The listing builds one solid part. Answer for the finished solid, in the listing's coordinates (mm). Face numbers are marked on the shaded views. A direction names the side the tool comes from. Give positions to 0.01 mm unless a question says otherwise; leave off trailing zeros. Loops run counter-clockwise (first coordinate to the right, second up) from the corner with the lowest first, then second, coordinate; pieces in that order, holes last. Notation, with made-up numbers: M 81,37.5 L 132,37.5 A27 cw 132,56.5 Z; hole C 12.25,-37 d11. An arc over 180 degrees is marked long. One line per item, written item: value. Start each with the question number.
Q1. Consider L1, parallel to Z at x = 50, y = 8.7 (3 decimals); L2, parallel to Z at x = 8.95, y = 1.5; L3, parallel to Z at x = 71.05, y = 10. Determine where each line is inside the solid, lowest interval first.
Q2. A cutting plane is placed at D-D, the plane y = -11. Determine the outline of the cut face in (x, z) (3 decimals), and give its area (3 significant figures).
Q3. A cutting plane is placed at A-A, the plane x = 28.95. Determine the outline of the cut face in (y, z).
Q4. Flat-ended cylindrical pins translate along their axes: pin 1 (8 mm diameter, centred on y = 12, z = -65.5, fed in from +X); pin 2 (3 mm diameter, centred on x = 37.5, z = -115, fed in from -Y); pin 3 (9.5 mm diameter, centred on y = 3, z = -75, fed in from -X); pin 4 (5 mm diameter, centred on x = 83, z = -26.5, fed in from -Y). Find the tip coordinate at first contact, or state that the pin passes through.
Q5. A cutting plane is placed at B-B, the plane z = -56.47. Determine the outline of the cut face in (x, y).
Q6. A cutting plane is placed at C-C, the plane z = -92. Determine the outline of the cut face in (x, y), and give its area (3 significant figures).
Q7. For the marked faces 1, 2 and 3, determine the directions among +Z, -Z, +X, -X, +Y, -Y from which every point of the face is accessible in a straight line to the end or side of a thin tool.
from build123d import *

# Parameters (mm, degrees)
SKETCH1_W                      = 100
SKETCH1_H                      = 37
BOSS_EXTRUDE1_DEPTH            = 6
M3_CLEARANCE_HOLE1_D           = 3.4
SKETCH31_W                     = 20
SKETCH31_H                     = 29.63
BOSS_EXTRUDE9_DEPTH            = 16
BOSS_EXTRUDE9_DEPTH_BACK       = 9
SKETCH32_W                     = 100
SKETCH32_H                     = 5
BOSS_EXTRUDE10_DEPTH           = 16
SKETCH33_R                     = 3
BOSS_EXTRUDE11_DEPTH           = 3
SKETCH34_W                     = 3
SKETCH34_H                     = 19.5
CUT_EXTRUDE1_DEPTH             = 101
CUT_EXTRUDE2_START             = -2.5
SKETCH35_W                     = 20
SKETCH35_H                     = 20.32
CUT_EXTRUDE2_DEPTH             = 19.5
SKETCH36_R                     = 2.5
CUT_EXTRUDE3_DEPTH             = 26
FILLET1_R                      = 5
SKETCH37_R                     = 3
SKETCH37_R_2                   = 2.5
BOSS_EXTRUDE12_DEPTH           = 6.5
BOSS_EXTRUDE12_DEPTH_BACK      = 2.5
CBORE_FOR_M5_SHCS1_D           = 5.5
CBORE_FOR_M5_SHCS1_CBORE_D     = 10
CBORE_FOR_M5_SHCS1_CBORE_DEPTH = 26
M5_CLEARANCE_HOLE1_D           = 5.5
FILLET3_R                      = 5
SKETCH48_W                     = 11.20158878
SKETCH48_H                     = 10
BOSS_EXTRUDE15_DEPTH           = 14


with BuildPart() as part:
    # Sketch1 → Boss-Extrude1 (new body)
    with BuildSketch(Plane(origin=(0, 0, 0), x_dir=(1, 0, 0), z_dir=(0, 1, 0))):
        with Locations((50, 18.5)):
            Rectangle(SKETCH1_W, SKETCH1_H)
    extrude(amount=BOSS_EXTRUDE1_DEPTH)

    # M3 Clearance Hole1 (through all)
    with Locations(Plane(origin=(0, 0, 0), x_dir=(-1, 0, 0), z_dir=(0, -1, 0))):
        with Locations((-8.95, 3.5), (-8.95, 28.5), (-28.95, 28.5), (-28.95, 3.5), (-71.05, 3.5), (-71.05, 28.5), (-91.05, 28.5), (-91.05, 3.5)):
            Hole(M3_CLEARANCE_HOLE1_D / 2)

    # Sketch31 → Boss-Extrude9 (add, two sides)
    with BuildSketch(Plane.XZ) as boss_extrude9_sk:
        with Locations((50, -51.815)):
            Rectangle(SKETCH31_W, SKETCH31_H)
    extrude(amount=BOSS_EXTRUDE9_DEPTH)
    extrude(boss_extrude9_sk.sketch, amount=-BOSS_EXTRUDE9_DEPTH_BACK)

    # Sketch32 → Boss-Extrude10 (add)
    with BuildSketch(Plane.XZ):
        with Locations((50, -34.5)):
            Rectangle(SKETCH32_W, SKETCH32_H)
    extrude(amount=BOSS_EXTRUDE10_DEPTH)

    # Sketch33 → Boss-Extrude11 (add)
    with BuildSketch(Plane(origin=(0, 6, 0), x_dir=(1, 0, 0), z_dir=(0, 1, 0))):
        Polygon((0, 37), (0, 0), (100, 0), (100, 37), (60, 37), (40, 37), align=None)
        with Locations((71.05, 3.5)):
            Circle(SKETCH33_R, mode=Mode.SUBTRACT)
        with Locations((71.05, 28.5)):
            Circle(SKETCH33_R, mode=Mode.SUBTRACT)
        with Locations((28.95, 3.5)):
            Circle(SKETCH33_R, mode=Mode.SUBTRACT)
        with Locations((28.95, 28.5)):
            Circle(SKETCH33_R, mode=Mode.SUBTRACT)
        with Locations((8.95, 28.5)):
            Circle(SKETCH33_R, mode=Mode.SUBTRACT)
        with Locations((8.95, 3.5)):
            Circle(SKETCH33_R, mode=Mode.SUBTRACT)
        with Locations((91.05, 3.5)):
            Circle(SKETCH33_R, mode=Mode.SUBTRACT)
        with Locations((91.05, 28.5)):
            Circle(SKETCH33_R, mode=Mode.SUBTRACT)
    extrude(amount=BOSS_EXTRUDE11_DEPTH)

    # Sketch34 → Cut-Extrude1 (cut, through all)
    with BuildSketch(Plane(origin=(100, 0, 0), x_dir=(0, 0, -1), z_dir=(1, 0, 0))):
        with Locations((37.5, -3.25)):
            Rectangle(SKETCH34_W, SKETCH34_H)
    extrude(amount=-CUT_EXTRUDE1_DEPTH, mode=Mode.SUBTRACT)

    # Sketch35 → Cut-Extrude2 (cut)
    with BuildSketch(Plane(origin=(0, 9, 0), x_dir=(1, 0, 0), z_dir=(0, 1, 0)).offset(CUT_EXTRUDE2_START)):
        with Locations((50, 56.47)):
            Rectangle(SKETCH35_W, SKETCH35_H)
    extrude(amount=-CUT_EXTRUDE2_DEPTH, mode=Mode.SUBTRACT)

    # Sketch36 → Cut-Extrude3 (cut, through all)
    with BuildSketch(Plane(origin=(0, 9, 0), x_dir=(1, 0, 0), z_dir=(0, 1, 0))):
        with Locations((50, 56.47)):
            Circle(SKETCH36_R)
    extrude(amount=-CUT_EXTRUDE3_DEPTH, mode=Mode.SUBTRACT)

    # Fillet1
    fillet1_edges = [part.edges().sort_by_distance(p)[0] for p in [
        (60, 7.75, -66.63),
        (40, 7.75, -66.63),
        (40, -14.5, -66.63),
        (60, -14.5, -66.63),
    ]]
    fillet(fillet1_edges, radius=FILLET1_R)

    # Sketch37 → Boss-Extrude12 (add, two sides)
    with BuildSketch(Plane(origin=(0, 9, 0), x_dir=(1, 0, 0), z_dir=(0, 1, 0))) as boss_extrude12_sk:
        Polygon((40, 37), (0, 37), (0, 0), (100, 0), (100, 37), (60, 37), (60, 137), (40, 137), align=None)
        with Locations((28.95, 3.5)):
            Circle(SKETCH37_R, mode=Mode.SUBTRACT)
        with Locations((8.95, 3.5)):
            Circle(SKETCH37_R, mode=Mode.SUBTRACT)
        with Locations((8.95, 28.5)):
            Circle(SKETCH37_R, mode=Mode.SUBTRACT)
        with Locations((28.95, 28.5)):
            Circle(SKETCH37_R, mode=Mode.SUBTRACT)
        with Locations((71.05, 28.5)):
            Circle(SKETCH37_R, mode=Mode.SUBTRACT)
        with Locations((91.05, 28.5)):
            Circle(SKETCH37_R, mode=Mode.SUBTRACT)
        with Locations((91.05, 3.5)):
            Circle(SKETCH37_R, mode=Mode.SUBTRACT)
        with Locations((71.05, 3.5)):
            Circle(SKETCH37_R, mode=Mode.SUBTRACT)
        with Locations((50, 56.47)):
            Circle(SKETCH37_R_2, mode=Mode.SUBTRACT)
    extrude(amount=BOSS_EXTRUDE12_DEPTH)
    extrude(boss_extrude12_sk.sketch, amount=-BOSS_EXTRUDE12_DEPTH_BACK)

    # CBORE for M5 SHCS1 (through all)
    with Locations(Plane(origin=(0, -16, 0), x_dir=(-1, 0, 0), z_dir=(0, -1, 0))):
        with Locations((-50, 127), (-50, 92)):
            CounterBoreHole(CBORE_FOR_M5_SHCS1_D / 2, CBORE_FOR_M5_SHCS1_CBORE_D / 2, CBORE_FOR_M5_SHCS1_CBORE_DEPTH)

    # M5 Clearance Hole1 (through all)
    with Locations(Plane(origin=(0, -16, 0), x_dir=(-1, 0, 0), z_dir=(0, -1, 0))):
        with Locations((-50, 42.655)):
            Hole(M5_CLEARANCE_HOLE1_D / 2)

    # Fillet3
    fillet3_edges = [part.edges().sort_by_distance(p)[0] for p in [
        (60, 11, -137),
        (40, 11, -137),
    ]]
    fillet(fillet3_edges, radius=FILLET3_R)

    # Sketch48 → Boss-Extrude15 (add)
    with BuildSketch(Plane.XZ):
        with Locations((50, -31)):
            Rectangle(SKETCH48_W, SKETCH48_H)
    extrude(amount=BOSS_EXTRUDE15_DEPTH)


solid = part.part
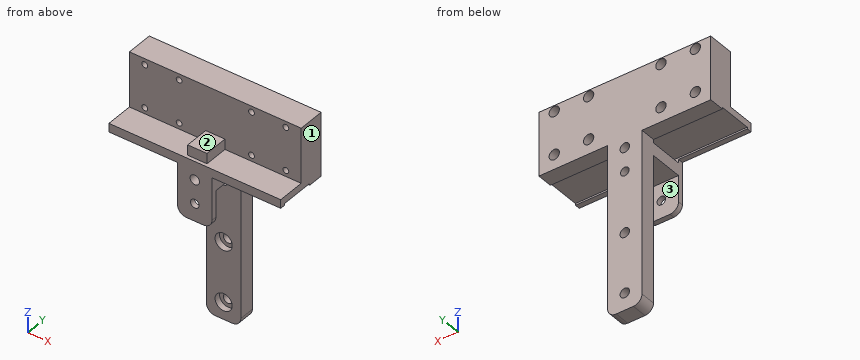
Answer block:
1. L1: -137 to -132, -122 to -97, -87 to -58.97, -53.97 to -45.405, -39.905 to 0
1. L2: -36 to -30.2, -26.8 to -5.2, -1.8 to 0
1. L3: -37 to -31.5, -25.5 to -6.5, -0.5 to 0
2. outline: M 0,-36 L 100,-36 L 100,-32 L 55.601,-32 L 55.601,-26 L 44.399,-26 L 44.399,-32 L 0,-32 Z; M 40,-46.31 L 60,-46.31 L 60,-39 L 40,-39 Z; hole C 50,-42.655 d5.5
2. area: 590 mm^2
3. outline: M -16,-37 L -13,-37 L -13,-36 L 6.5,-36 L 6.5,-37 L 15.5,-37 L 15.5,-31.5 L 6,-31.5 L 6,-30.2 L 0,-30.2 L 0,-32 L -16,-32 Z; M 0,-26.8 L 6,-26.8 L 6,-25.5 L 15.5,-25.5 L 15.5,-6.5 L 6,-6.5 L 6,-5.2 L 0,-5.2 Z; M 0,-1.8 L 6,-1.8 L 6,-0.5 L 15.5,-0.5 L 15.5,0 L 0,0 Z
4. pin 1: x = 60
4. pin 2: through
4. pin 3: x = 40
4. pin 4: y = 0
5. outline: M 40,-16 L 47.5,-16 L 47.5,-13 L 40,-13 Z; M 40,6.5 L 47.5,6.5 L 47.5,15.5 L 40,15.5 Z; M 52.5,-16 L 60,-16 L 60,-13 L 52.5,-13 Z; M 52.5,6.5 L 60,6.5 L 60,15.5 L 52.5,15.5 Z
6. outline: M 40,6.5 L 45,6.5 L 45,10 L 47.25,10 L 47.25,15.5 L 40,15.5 Z; M 52.75,10 L 55,10 L 55,6.5 L 60,6.5 L 60,15.5 L 52.75,15.5 Z
6. area: 115 mm^2
7. face 1: +Z, -Z, +X, +Y, -Y
7. face 2: +Z, +X, -X, -Y
7. face 3: -Z, +X, -X
